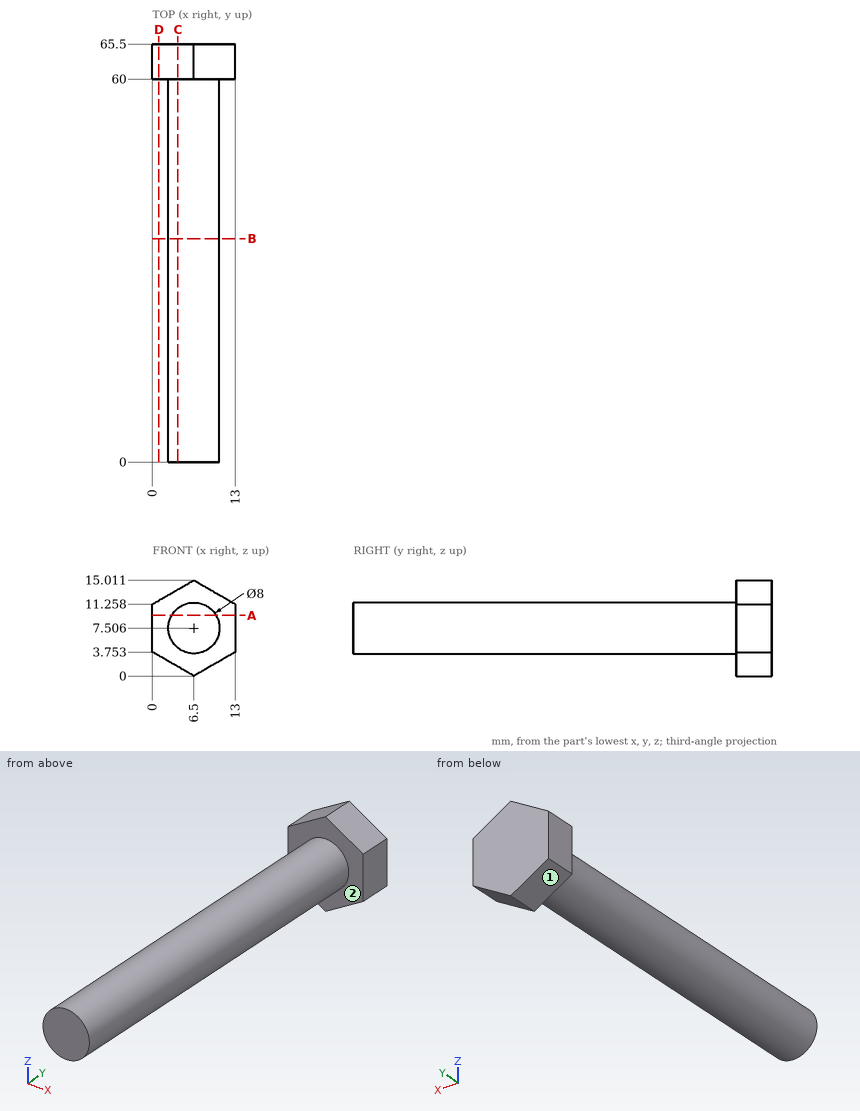
Geometry check sheet. Reference: drawing and pictorial views, mm from the part's lowest x, y, z. A direction names the side the tool comes from. Give positions to 0.01 mm unless a question says otherwise; leave off trailing zeros. Loops run counter-clockwise (first coordinate to the right, second up) from the corner with the lowest first, then second, coordinate; pieces in that order, holes last. Notation, with made-up numbers: (-11, 25.5) - (4, 25.5) arc R20 ccw to (4, 63.5) - close; hole circle Ø6 at (-29.5, 18.5). An arc over 180 degrees is marked (long way). Use CSV: the item, a comma, the result in double quotes. Start each with the question number.
Q1. Scan lines: probe 1 along Y at (x, z) = (7.75, 1.5); probe 2 along X at (y, z) = (48.5, 4.25) (1 decimal); probe 3 along Z at (x, y) = (7.5, 26.5). Record each from-to range of solid material in increasing order. Write a range as from..to.
Q2. Access from +Z, -Z, +X, -X, +Y, -Y to the whole of each face (thin tool, end or side, straight path). Record for the marked faces 1 and 2.
Q3. Go/stop test with flat-tipped pins: pin 1 Ø3 at (x, y) = (7, 52) entering from +Z; pin 2 Ø1 at (y, z) = (14, 11.5) entering from +X (1 decimal); pin 3 Ø4 at (y, z) = (47, 6) entering from +X. Record where each tip stops, or that it passes through.
Q4. Section check C-C, the plane x = 4. Record the cut outline in (y, z).
Q5. Section check A-A, the plane z = 9.5. Record the cut outline in (x, y).
Q6. Section check D-D, the plane x = 1. Record the cut outline in (y, z) (1 decimal).
Q7. Section check B-B, the plane y = 35. Record the cut outline in (x, z) (1 decimal).
Findings below:
1,probe 1,"y = 60..65.5"
1,probe 2,"x = 4.2..8.8"
1,probe 3,"z = 3.63..11.38"
2,face 1,"-Z, -X, +Y, -Y"
2,face 2,"-Y"
3,pin 1,"stops at z = 11.51"
3,pin 2,"stops at x = 8.4"
3,pin 3,"stops at x = 10.5"
4,outline,"(0, 4.38) - (60, 4.38) - (60, 1.44) - (65.5, 1.44) - (65.5, 13.57) - (60, 13.57) - (60, 10.63) - (0, 10.63) - close"
5,outline,"(0, 60) - (3.03, 60) - (3.03, 0) - (9.97, 0) - (9.97, 60) - (13, 60) - (13, 65.5) - (0, 65.5) - close"
6,outline,"(60, 3.2) - (65.5, 3.2) - (65.5, 11.8) - (60, 11.8) - close"
7,outline,"circle Ø8 at (6.5, 7.5)"
